from build123d import *

# Parameters (mm, degrees)
SM_BASE_FLANGE_1_DEPTH = 45
SKETCH_6_R             = 3.5
CUT_EXTRUDE_1_DEPTH    = 10
SKETCH_7_R             = 3.5
CUT_EXTRUDE_2_DEPTH    = 10


# Sheet-metal steps are written as plain solids
with BuildPart() as part:
    # Sketch 1 → Базовая кромка1 (new body)
    with BuildSketch(Plane.XY):
        with BuildLine():
            Line((-48.5, 428.5), (-48.5, 401.5))
            ThreePointArc((-48.5, 401.5), (-48.060660172, 400.439339828), (-47, 400))
            Line((-47, 400), (-3, 400))
            ThreePointArc((-3, 400), (-0.878679656, 399.121320344), (0, 397))
            Line((0, 397), (0, 3))
            ThreePointArc((0, 3), (-0.878679656, 0.878679656), (-3, 0))
            Line((-3, 0), (-65, 0))
            Line((-65, 0), (-65, 1.5))
            Line((-65, 1.5), (-3, 1.5))
            ThreePointArc((-3, 1.5), (-1.939339828, 1.939339828), (-1.5, 3))
            Line((-1.5, 3), (-1.5, 397))
            ThreePointArc((-1.5, 397), (-1.939339828, 398.060660172), (-3, 398.5))
            Line((-3, 398.5), (-47, 398.5))
            ThreePointArc((-47, 398.5), (-49.121320344, 399.378679656), (-50, 401.5))
            Line((-50, 401.5), (-50, 428.5))
            Line((-50, 428.5), (-48.5, 428.5))
        make_face()
    extrude(amount=-SM_BASE_FLANGE_1_DEPTH)

    # Эскиз6 → Вырез-Вытянуть1 (cut)
    with BuildSketch(Plane(origin=(0, 1.5, 0), x_dir=(1, 0, 0), z_dir=(0, 1, 0))):
        with Locations(Location((-59.5, 35, 0), (0, 0, 180))):
            Circle(SKETCH_6_R)
        with Locations(Location((-59.5, 10, 0), (0, 0, 180))):
            Circle(SKETCH_6_R)
    extrude(amount=-CUT_EXTRUDE_1_DEPTH, mode=Mode.SUBTRACT)

    # Эскиз7 → Вырез-Вытянуть2 (cut)
    with BuildSketch(Plane.ZY.offset(50)):
        with Locations((-35, 412.5)):
            Circle(SKETCH_7_R)
        with Locations((-10, 412.5)):
            Circle(SKETCH_7_R)
    extrude(amount=-CUT_EXTRUDE_2_DEPTH, mode=Mode.SUBTRACT)


solid = part.part
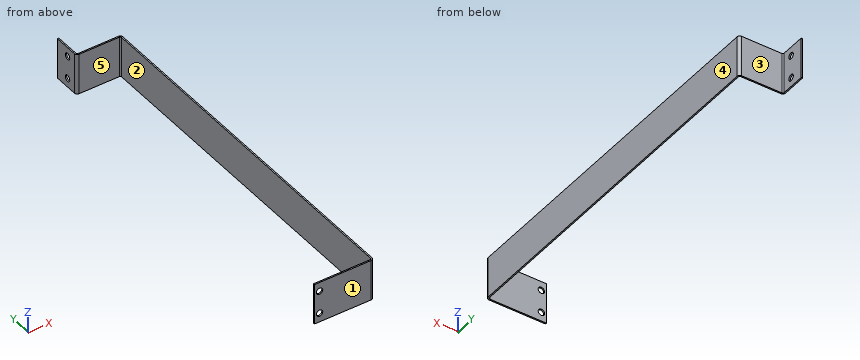
Input: part model. Units: mm. Frame: model coordinates. Face numbers are marked on the shaded views. A direction names the side the tool comes from. Give positions to 0.01 mm unless a question says otherwise; leave off trailing zeros. Loops run counter-clockwise (first coordinate to the right, second up) from the corner with the lowest first, then second, coordinate; pieces in that order, holes last. Notation, with made-up numbers: (28.5, 21) -> (32.5, 21) arc R27 cw to (32.5, 42) -> close; hole circle Ø8 at (3, -19.75). An arc over 180 degrees is marked (long way). Answer as a JSON object with one key per item and string values. Group by question number.
Item 1: Cut plane D-D, the plane y = 269. Return the cut outline in (x, z).
Item 2: Pin query (flat end, axial travel): P1, Ø13.5, axis at y = 417, z = -24, coming from the +X side; P2, Ø12, axis at y = 296.5, z = -33.5, coming from the -X side; P3, Ø10, axis at x = -25.5, z = -27, coming from the +Y side. Return the tip coordinate at first contact, or that it passes through.
Item 3: Line query: probe 1 along Z at (x, y) = (-59, 1); probe 2 along Y at (x, z) = (-25.5, -19); probe 3 along Y at (x, z) = (-49.7, -10). Output: solid intervals per line, ascending.
Item 4: Cut plane A-A, the plane x = -26.5. Return the cut outline in (y, z), and give its area (3 significant figures).
Item 5: Pull-direction query (Y, two-part tool) for the marked faces 3, 4 and 5; classes: released by +Y, released by -Y, zero draft, split by the parting line, or undercut.
Item 6: Cut plane B-B, the plane z = -10. Return the cut outline in (x, y), and give its area (3 significant figures).
Item 7: Cut plane C-C, the plane x = -59.5. Return the cut outline in (y, z), and give its area (3 significant figures).
Item 8: Reachability of the marked faces 1 and 2 from +Z, -Z, +X, -X, +Y, -Y: full face, straight path, thin tool, end or side. Return the list, or none.
Checks:
{
 "1": {"outline": "(-1.5, -45) -> (0, -45) -> (0, 0) -> (-1.5, 0) -> close"},
 "2": {"P1": "stops at x = -48.5", "P2": "stops at x = -1.5", "P3": "stops at y = 400"},
 "3": {"probe 1": "z = -45 to -38.46, -31.54 to -13.46, -6.54 to 0", "probe 2": "y = 0 to 1.5, 398.5 to 400", "probe 3": "y = 0 to 1.5, 400.19 to 409, 416 to 428.5"},
 "4": {"outline": "(0, -45) -> (1.5, -45) -> (1.5, 0) -> (0, 0) -> close; (398.5, -45) -> (400, -45) -> (400, 0) -> (398.5, 0) -> close", "area": "135 mm²"},
 "5": {"face 3": "released by +Y", "face 4": "zero draft", "face 5": "undercut"},
 "6": {"outline": "(-65, 0) -> (-63, 0) -> (-63, 1.5) -> (-65, 1.5) -> close; (-56, 0) -> (-3, 0) arc R3 ccw to (0, 3) -> (0, 397) arc R3 ccw to (-3, 400) -> (-47, 400) arc R1.5 cw to (-48.5, 401.5) -> (-48.5, 409) -> (-50, 409) -> (-50, 401.5) arc R3 ccw to (-47, 398.5) -> (-3, 398.5) arc R1.5 cw to (-1.5, 397) -> (-1.5, 3) arc R1.5 cw to (-3, 1.5) -> (-56, 1.5) -> close; (-50, 416) -> (-48.5, 416) -> (-48.5, 428.5) -> (-50, 428.5) -> close", "area": "785 mm²"},
 "7": {"outline": "(0, -45) -> (1.5, -45) -> (1.5, -38.5) -> (0, -38.5) -> close; (0, -31.5) -> (1.5, -31.5) -> (1.5, -13.5) -> (0, -13.5) -> close; (0, -6.5) -> (1.5, -6.5) -> (1.5, 0) -> (0, 0) -> close", "area": "46.5 mm²"},
 "8": {"face 1": "+Z, -Z, +X, -X, -Y", "face 2": "+Z, -Z, -X"}
}
